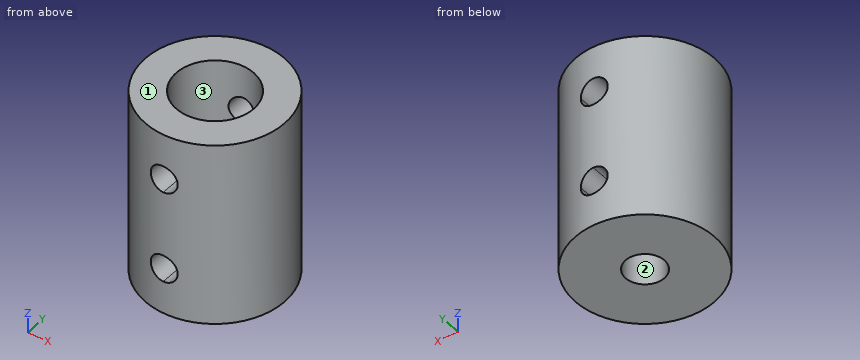
from build123d import *

# Parameters (mm, degrees)
F0_R          = 9
F1_DEPTH      = 24
F2_R          = 5
F3_DEPTH      = 10
F4_R          = 2.5
F5_DEPTH      = 10
F7_DEPTH      = 25
F7_DEPTH_BACK = 25


with BuildPart() as f1:
    # F0 (on Top) → F1 (new body)
    with BuildSketch(Plane.XY):
        Circle(F0_R)
    extrude(amount=F1_DEPTH)

    # F2 (on face) → F3 (cut)
    with BuildSketch(Plane.XY.offset(24)):
        Circle(F2_R)
    extrude(amount=-F3_DEPTH, mode=Mode.SUBTRACT)

    # F4 (on Top) → F5 (cut)
    with BuildSketch(Plane.XY):
        Circle(F4_R)
    extrude(amount=F5_DEPTH, mode=Mode.SUBTRACT)

    # F6 (on Front) → F7 (cut, two sides)
    with BuildSketch(Plane.XZ) as f7_sk:
        with BuildLine():
            ThreePointArc((0, 7.75), (-1.75, 6), (0, 4.25))
            Line((0, 4.25), (0, 6))
            Line((0, 6), (0, 7.75))
        make_face()
        with BuildLine():
            ThreePointArc((1.75, 18), (-1.2374368671, 19.2374368671), (0, 16.25))
            ThreePointArc((0, 16.25), (1.2374368671, 16.7625631329), (1.75, 18))
        make_face()
        with BuildLine():
            Line((0, 6), (0, 4.25))
            ThreePointArc((0, 4.25), (1.2374368671, 4.7625631329), (1.75, 6))
            ThreePointArc((1.75, 6), (1.2374368671, 7.2374368671), (0, 7.75))
            Line((0, 7.75), (0, 6))
        make_face()
    extrude(amount=-F7_DEPTH, mode=Mode.SUBTRACT)
    extrude(f7_sk.sketch, amount=F7_DEPTH_BACK, mode=Mode.SUBTRACT)


solid = f1.part
Read the model definition and answer for the solid it produces. Units are mm, in the model's axes. Face numbers are marked on the shaded views. A direction names the side the tool comes from. Coordinates: 2 decimals unless noted, no trailing zeros. Write each loop counter-clockwise with the first axis right and the second up, starting at its lowest first coordinate (ties: lowest second). Pieces come first, ordered by that corner, then holes. Notation, with made-up numbers: (15.25, 0.5) -> (33.25, 0.5) arc R19 ccw to (33.25, 33.5) -> close; hole circle Ø2 at (-7, 68). An arc over 180 degrees is marked (long way). Return JSON: item names as keys, results as strings.
(1) The part is cut by section D-D on y = 4. Give the vertices of the cut face in (x, z), then the cut area to 3 significant figures.
Answers below:
{"outline": "(-8.06, 0) -> (8.06, 0) -> (8.06, 24) -> (3, 24) -> (3, 14) -> (-3, 14) -> (-3, 24) -> (-8.06, 24) -> close; hole circle Ø3.5 at (0, 6)", "area": "317 mm^2"}
(2) The part is cut by section A-A on x = 0.5. Give the vertices of the cut face in (y, z), then the cut area to 3 significant figures.
Answers below:
{"outline": "(-8.99, 0) -> (-2.45, 0) -> (-2.45, 4.32) -> (-8.99, 4.32) -> close; (-8.99, 7.68) -> (-2.45, 7.68) -> (-2.45, 10) -> (2.45, 10) -> (2.45, 7.68) -> (8.99, 7.68) -> (8.99, 16.32) -> (4.97, 16.32) -> (4.97, 14) -> (-4.97, 14) -> (-4.97, 16.32) -> (-8.99, 16.32) -> close; (-8.99, 19.68) -> (-4.97, 19.68) -> (-4.97, 24) -> (-8.99, 24) -> close; (2.45, 0) -> (8.99, 0) -> (8.99, 4.32) -> (2.45, 4.32) -> close; (4.97, 19.68) -> (8.99, 19.68) -> (8.99, 24) -> (4.97, 24) -> close", "area": "212 mm^2"}
(3) The part is cut by section B-B on y = 0. Give the vertices of the cut face in (x, z), then the cut area to 3 significant figures.
Answers below:
{"outline": "(-9, 0) -> (-2.5, 0) -> (-2.5, 10) -> (2.5, 10) -> (2.5, 0) -> (9, 0) -> (9, 24) -> (5, 24) -> (5, 14) -> (-5, 14) -> (-5, 24) -> (-9, 24) -> close", "area": "282 mm^2"}
(4) Each of these flat-tipped pins is pushed along its axis until it touches: P1, Ø8, axis at y = -5.5, z = 13, coming from the -X side; P2, Ø3, axis at x = 5.5, y = -6, coming from the -Z side; P3, Ø10, axis at y = 5.5, z = 21, coming from the +X side; P4, Ø3, axis at x = 6.5, z = 11, coming from the +Y side. Where does it stop, or does it pass through?
Answers below:
{"P1": "x = -8.87", "P2": "z = 0", "P3": "x = 8.99", "P4": "y = 7.48"}
(5) The part is cut by section C-C on z = 18.5. Give the vertices of the cut face in (x, y), then the cut area to 3 significant figures.
Answers below:
{"outline": "(-1.68, -8.84) -> (-1.68, -4.71) arc R5 cw to (-1.68, 4.71) -> (-1.68, 8.84) arc R9 ccw to start; (1.68, -8.84) arc R9 ccw to (1.68, 8.84) -> (1.68, 4.71) arc R5 cw to (1.68, -4.71) -> close", "area": "149 mm^2"}
(6) Which of the six approach directions +Z, -Z, +X, -X, +Y, -Y give full straight-line access (tool end or side, diameter ignored) to the marked faces 1, 2 and 3?
Answers below:
{"face 1": "+Z, +X, -X, +Y, -Y", "face 2": "-Z", "face 3": "+Z"}
(7) Consider line 1 along Z through (x, y) = (1.25, 7.75); line 2 along Y through (x, z) = (0, 21.75); line 3 along X through (y, z) = (-2.5, 16.25). Determine where each line is inside the solid, lowest interval first. Write a range as from..to.
Answers below:
{"line 1": "0..4.78, 7.22..16.78, 19.22..24", "line 2": "-9..-5, 5..9", "line 3": "-8.65..-4.33, 4.33..8.65"}
